Geometry: final body of the model. Coordinates: model frame, mm. A direction names the side the tool comes from. Give positions to 0.01 mm unless a question says otherwise; leave off trailing zeros. Order: outer loops, then holes, each group sorted by start corner. A loop starts at its lowest first (then second) coordinate and runs counter-clockwise, first axis right, second up. Notation, with made-up numbers: (75, -14.5) - (84, -14.5) arc R38 ccw to (84, 24.5) - close; hole circle Ø9 at (-22, -26.5). An arc over 180 degrees is marked (long way). Use one line per item in the form item = value.
from build123d import *

# Parameters (mm, degrees)
F0_W           = 50
F0_H           = 3
F1_DEPTH       = 12
F3_DEPTH       = 45
F5_DEPTH       = 120.001
F6_R           = 12
F6_R_2         = 1.65
F7_DEPTH       = 25
F9_D           = 3.7973
F9_CSINK_D     = 7.7978
F9_CSINK_ANGLE = 82
F10_W          = 1
F10_H          = 5
F11_DEPTH      = 0.4
F13_END_RADIUS = 35
F13_REACH      = 75.7248075794
F14_END_RADIUS = 35
F14_REACH      = 75.7248075794
F15_DEPTH      = 25


with BuildPart() as f1:
    # F0 (on Front) → F1 (new body)
    with BuildSketch(Plane.XZ):
        with BuildLine():
            Line((22.8227958083, 19.723181963), (-27.1772041917, 19.723181963))
            ThreePointArc((-27.1772041917, 19.723181963), (-37.4284668502, -5.0255553786), (-62.1772041917, -15.276818037))
            Line((-62.1772041917, -15.276818037), (-62.1772041917, -29.276818037))
            Line((-62.1772041917, -29.276818037), (57.8227958083, -29.276818037))
            Line((57.8227958083, -29.276818037), (57.8227958083, -15.276818037))
            ThreePointArc((57.8227958083, -15.276818037), (33.0740584668, -5.0255553786), (22.8227958083, 19.723181963))
        make_face()
        with Locations((-2.1772041917, 21.223181963)):
            Rectangle(F0_W, F0_H)
    extrude(amount=F1_DEPTH)

    # F2 (on face) → F3 (join)
    with BuildSketch(Plane.XZ.offset(12)):
        with BuildLine():
            Line((-25.1772041917, 19.723181963), (-27.1772041917, 19.723181963))
            ThreePointArc((-27.1772041917, 19.723181963), (-37.4284668502, -5.0255553786), (-62.1772041917, -15.276818037))
            Line((-62.1772041917, -15.276818037), (-62.1772041917, -29.276818037))
            Line((-62.1772041917, -29.276818037), (-60.1772041917, -29.276818037))
            Line((-60.1772041917, -29.276818037), (-60.1772041917, -17.2227244409))
            ThreePointArc((-60.1772041917, -17.2227244409), (-35.3164521546, -5.722839337), (-25.1772041917, 19.723181963))
        make_face()
        Polygon((-27.1772041917, 22.723181963), (-27.1772041917, 19.723181963), (-25.1772041917, 19.723181963), (20.8227958083, 19.723181963), (22.8227958083, 19.723181963), (22.8227958083, 22.723181963), align=None)
        with BuildLine():
            Line((22.8227958083, 19.723181963), (20.8227958083, 19.723181963))
            ThreePointArc((20.8227958083, 19.723181963), (30.9620437712, -5.722839337), (55.8227958083, -17.2227244409))
            Line((55.8227958083, -17.2227244409), (55.8227958083, -29.276818037))
            Line((55.8227958083, -29.276818037), (57.8227958083, -29.276818037))
            Line((57.8227958083, -29.276818037), (57.8227958083, -15.276818037))
            ThreePointArc((57.8227958083, -15.276818037), (33.0740584668, -5.0255553786), (22.8227958083, 19.723181963))
        make_face()
    extrude(amount=F3_DEPTH)

    # F4 (on face) → F5 (cut, through all)
    with BuildSketch(Plane(origin=(-62.1772041917, 0, 0), x_dir=(0, -1, 0), z_dir=(-1, 0, 0))):
        with BuildLine():
            Line((57, -15.276818037), (57, 19.723181963))
            ThreePointArc((57, 19.723181963), (26.3280584166, 2.7280262742), (12, -29.276818037))
            Line((12, -29.276818037), (57, -29.276818037))
            Line((57, -29.276818037), (57, -15.276818037))
        make_face()
    extrude(amount=-F5_DEPTH, mode=Mode.SUBTRACT)

    # F6 (on face) → F7 (cut)
    with BuildSketch(Plane.XY.offset(22.723181963)):
        with Locations((-2.1772041917, -35.85)):
            Circle(F6_R)
        with Locations((-17.6772041917, -51.35)):
            Circle(F6_R_2)
        with Locations((-17.6772041917, -20.35)):
            Circle(F6_R_2)
        with Locations((13.3227958083, -51.35)):
            Circle(F6_R_2)
        with Locations((13.3227958083, -20.35)):
            Circle(F6_R_2)
    extrude(amount=-F7_DEPTH, mode=Mode.SUBTRACT)

    # F9 (through all)
    with Locations(Plane.XZ.offset(12)):
        with Locations((-30.1772041917, -23.2497712389), (25.8227958083, -23.2497712389)):
            CounterSinkHole(F9_D / 2, F9_CSINK_D / 2, counter_sink_angle=F9_CSINK_ANGLE)

    # F10 (on face) → F11 (join)
    with BuildSketch(Plane.XY.offset(22.723181963)):
        with Locations((-2.1772041917, -2.5)):
            Rectangle(F10_W, F10_H)
    extrude(amount=F11_DEPTH)

    f13_end = (Plane(origin=(-62.1772041917, -28.5, 19.723181963), x_dir=(0, 0, 1), z_dir=(0, 1, 0)) * Cylinder(F13_END_RADIUS, 437.0700631752, mode=Mode.PRIVATE)).faces().sort_by_distance((-37.4284668502, -0.7549172174, -5.0255553786))[0]
    # F12 (on face) → F13 (join, up to the whole of a round face its end follows)
    with BuildSketch(Plane(origin=(0, 0, -29.276818037), x_dir=(1, 0, 0), z_dir=(0, 0, -1))):
        with BuildLine():
            Line((-62.1772041917, 24), (-62.1772041917, 12))
            Line((-62.1772041917, 12), (-60.1772041917, 12))
            Line((-60.1772041917, 12), (-56.2272041917, 12))
            ThreePointArc((-56.2272041917, 12), (-52.1772041917, 16.05), (-48.1272041917, 12))
            Line((-48.1272041917, 12), (-42.1772041917, 12))
            Line((-42.1772041917, 12), (-42.1772041917, 24))
            Line((-42.1772041917, 24), (-62.1772041917, 24))
        make_face()
        with BuildLine():
            Line((-56.2272041917, 12), (-48.1272041917, 12))
            ThreePointArc((-48.1272041917, 12), (-52.1772041917, 16.05), (-56.2272041917, 12))
        make_face()
    f13_long = extrude(amount=-F13_REACH, mode=Mode.PRIVATE)
    add(split(f13_long, bisect_by=f13_end, keep=Keep.TOP, mode=Mode.PRIVATE))

    f14_end = (Plane(origin=(57.8227958083, -28.5, 19.723181963), x_dir=(0, 0, 1), z_dir=(0, 1, 0)) * Cylinder(F14_END_RADIUS, 437.0700631752, mode=Mode.PRIVATE)).faces().sort_by_distance((33.0740584668, -0.7549172174, -5.0255553786))[0]
    # F12 (on face) → F14 (join, up to the whole of a round face its end follows)
    with BuildSketch(Plane(origin=(0, 0, -29.276818037), x_dir=(1, 0, 0), z_dir=(0, 0, -1))):
        with BuildLine():
            Line((37.8227958083, 24), (37.8227958083, 12))
            Line((37.8227958083, 12), (43.7727958083, 12))
            ThreePointArc((43.7727958083, 12), (47.8227958083, 16.05), (51.8727958083, 12))
            Line((51.8727958083, 12), (55.8227958083, 12))
            Line((55.8227958083, 12), (57.8227958083, 12))
            Line((57.8227958083, 12), (57.8227958083, 24))
            Line((57.8227958083, 24), (37.8227958083, 24))
        make_face()
        with BuildLine():
            Line((51.8727958083, 12), (43.7727958083, 12))
            ThreePointArc((43.7727958083, 12), (47.8227958083, 7.95), (51.8727958083, 12))
        make_face()
    f14_long = extrude(amount=-F14_REACH, mode=Mode.PRIVATE)
    add(split(f14_long, bisect_by=f14_end, keep=Keep.TOP, mode=Mode.PRIVATE))

    # F12 (on face) → F15 (cut)
    with BuildSketch(Plane(origin=(0, 0, -29.276818037), x_dir=(1, 0, 0), z_dir=(0, 0, -1))):
        with BuildLine():
            Line((-56.2272041917, 12), (-48.1272041917, 12))
            ThreePointArc((-48.1272041917, 12), (-52.1772041917, 16.05), (-56.2272041917, 12))
        make_face()
        with BuildLine():
            ThreePointArc((-56.2272041917, 12), (-52.1772041917, 7.95), (-48.1272041917, 12))
            Line((-48.1272041917, 12), (-56.2272041917, 12))
        make_face()
        with BuildLine():
            Line((51.8727958083, 12), (43.7727958083, 12))
            ThreePointArc((43.7727958083, 12), (47.8227958083, 7.95), (51.8727958083, 12))
        make_face()
        with BuildLine():
            ThreePointArc((51.8727958083, 12), (47.8227958083, 16.05), (43.7727958083, 12))
            Line((43.7727958083, 12), (51.8727958083, 12))
        make_face()
    extrude(amount=-F15_DEPTH, mode=Mode.SUBTRACT)


solid = f1.part
(1) Ray query, line 1 along X through (y, z) = (-51, 20); line 2 along Z through (x, y) = (-53.5, -3.5); line 3 along X through (y, z) = (-47.5, 19). Return the intervals inside material, ascending.
Computed values:
line_1 = -27.18 to -19.29, -16.06 to 11.71, 14.94 to 22.82
line_2 = -29.28 to -14.18
line_3 = -27.18 to -25.18, 20.83 to 22.83
(2) Cut plane B-B on y = -35.85. Output: boundary loops of the cut face in (x, z), plus the area to 3 significant figures.
Computed values:
outline = (-28.29, 10.98) - (-26.23, 10.98) arc R37 ccw to (-25.18, 19.72) - (-14.18, 19.72) - (-14.18, 22.72) - (-27.18, 22.72) - (-27.18, 19.72) arc R35 cw to start; (9.82, 19.72) - (20.82, 19.72) arc R37 ccw to (21.87, 10.98) - (23.93, 10.98) arc R35 cw to (22.82, 19.72) - (22.82, 22.72) - (9.82, 22.72) - close
area = 113 mm²
(3) Cut plane D-D on z = -7.5. Output: boundary loops of the cut face in (x, y), plus the area to 3 significant figures.
Computed values:
outline = (-40.18, -18.89) - (-37.12, -18.89) - (-37.12, -12) - (32.76, -12) - (32.76, -18.89) - (35.83, -18.89) - (35.83, 0) - (-40.18, 0) - close
area = 954 mm²
(4) Pull-direction query (X, two-part tool) for faces 1 (the face through (-62.177, -12, -22)), 2 (the face through (-3.739, -23.952, 21.244)), 3 (the face through (-3, 0, -9)); classes: released by +X, released by -X, zero draft, split by the parting line, or undercut.
Computed values:
face_1 = released by -X
face_2 = undercut
face_3 = zero draft
(5) Contact query for flat-ended pins moving along their axis: pin 1 Ø4.5 at (x, y) = (13.32, -51.35) entering from -Z; pin 2 Ø4 at (x, y) = (13.32, -20.35) entering from +Z; pin 3 Ø2 at (x, y) = (-17.68, -20.35) entering from +Z; pin 4 Ø6 at (x, z) = (-11.5, -1.5) entering from -Y. Output: stop coordinate, or through.
Computed values:
pin_1 = 19.72
pin_2 = 22.72
pin_3 = through
pin_4 = -12
(6) Cut plane C-C on y = -20.35. Output: boundary loops of the cut face in (x, z), plus the area to 3 significant figures.
Computed values:
outline = (-62.18, -29.28) - (-42.18, -29.28) - (-42.18, -9) arc R35 cw to (-62.18, -15.28) - close; (-37.47, -5.07) - (-34.71, -5.07) arc R37 ccw to (-25.18, 19.72) - (-19.33, 19.72) - (-19.33, 22.72) - (-27.18, 22.72) - (-27.18, 19.72) arc R35 cw to start; (-16.03, 19.72) - (11.67, 19.72) - (11.67, 22.72) - (-16.03, 22.72) - close; (14.97, 19.72) - (20.82, 19.72) arc R37 ccw to (30.36, -5.07) - (33.12, -5.07) arc R35 cw to (22.82, 19.72) - (22.82, 22.72) - (14.97, 22.72) - close; (37.82, -29.28) - (57.82, -29.28) - (57.82, -15.28) arc R35 cw to (37.82, -9) - close
area = 880 mm²
(7) Cut plane A-A on x = -12.5. Output: boundary loops of the cut face in (y, z), plus the area to 3 significant figures.
Computed values:
outline = (-57, 19.72) - (-41.97, 19.72) - (-41.97, 22.72) - (-57, 22.72) - close; (-29.73, 19.72) - (-12, 19.72) - (-12, -29.28) - (0, -29.28) - (0, 22.72) - (-29.73, 22.72) - close
area = 722 mm²
(8) Reachability of faces 4 (the face through (22.823, -28, 21)), 5 (the face through (-3, -57, 21)), 6 (the face through (-42.177, -18, -19)) from +Z, -Z, +X, -X, +Y, -Y: full face, straight path, thin tool, end or side. Return the list, or none.
Computed values:
face_4 = +Z, +X, +Y, -Y
face_5 = +Z, -Z, +X, -X, -Y
face_6 = -Z, -Y
